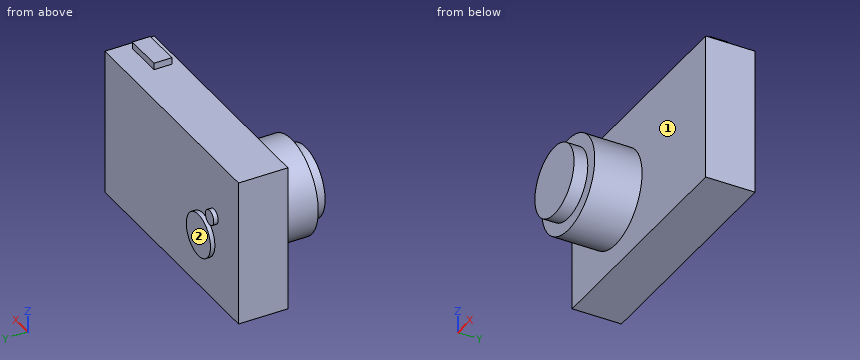
```python
from build123d import *

# Parameters (mm, degrees)
F0_W      = 180.9290349483
F0_H      = 111.6445362568
F1_DEPTH  = 25.4
F2_R      = 35.8615179987
F3_DEPTH  = 35.814
F4_R      = 26.5022456756
F5_DEPTH  = 10.414
F6_W      = 29.163653031
F6_H      = 13.6000299826
F7_DEPTH  = 5.08
F8_DEPTH  = 11.938
F10_R     = 16.3527851641
F10_R_2   = 5.6386158943
F11_DEPTH = 3.302


with BuildPart() as f1:
    # F0 (on Front) → F1 (new body)
    with BuildSketch(Plane.XZ):
        with Locations((-25.5821794271, -14.9854421616)):
            Rectangle(F0_W, F0_H)
    extrude(amount=F1_DEPTH)

    # F2 (on face) → F3 (join)
    with BuildSketch(Plane.XZ.offset(25.4)):
        with Locations((-57.2519302368, -18.0181078613)):
            Circle(F2_R)
    extrude(amount=F3_DEPTH)

    # F4 (on face) → F5 (join)
    with BuildSketch(Plane.XZ.offset(61.214)):
        with Locations((-57.2519302368, -18.0181078613)):
            Circle(F4_R)
    extrude(amount=F5_DEPTH)

    # F6 (on face) → F7 (join)
    with BuildSketch(Plane.XY.offset(40.8368259668)):
        with Locations((44.361977838, -12.2991851531)):
            Rectangle(F6_W, F6_H)
    extrude(amount=F7_DEPTH)

    # F8 (add): a face of the model
    f8_faces = [f1.faces().sort_by_distance(p)[0] for p in [
        (-25.5821794271, 0, -14.9854421616),
    ]]
    extrude(f8_faces, amount=F8_DEPTH)

    # F10 (on face) → F11 (join)
    with BuildSketch(Plane(origin=(0, 11.938, 0), x_dir=(-1, 0, 0), z_dir=(0, 1, 0))):
        with Locations((67.5977021456, -27.2572916001)):
            Circle(F10_R)
        with Locations((82.7291309834, -4.6637952328)):
            Circle(F10_R_2)
    extrude(amount=F11_DEPTH)


solid = f1.part
```
Source: CAD feature listing. Evaluate the final solid. Frame: model axes, mm. Face numbers are marked on the shaded views. A direction names the side the tool comes from. Give positions to 0.01 mm unless a question says otherwise; leave off trailing zeros. Loops run counter-clockwise (first coordinate to the right, second up) from the corner with the lowest first, then second, coordinate; pieces in that order, holes last. Notation, with made-up numbers: (54, 1) -> (103, 1) arc R22 ccw to (103, 35) -> close; hole circle Ø4 at (-6.5, -24.75). An arc over 180 degrees is marked (long way). Use a Markdown table: item, result. Add a question column.
(1) Access query for the marked faces 1 and 2. Directions: +Z, -Z, +X, -X, +Y, -Y. A direction counts if a zero-diameter tool reaches every point of the face in a straight line with its end or side. Return the directions, or none.
(2) Section query C-C (z = 32.5). Output: boundary loops of the cut face in (x, y).
(3) Section query A-A (x = 45). Output: boundary loops of the cut face in (y, z), then the cut area to 3 significant figures.
(4) First-contact query: pin 1 Ø2 at (x, z) = (-81.5, -2.5) entering from -Y; pin 2 Ø18.5 at (x, y) = (9, -2.5) entering from +Z; pin 3 Ø1.5 at (y, z) = (-12.5, 42.5) entering from +X. Flat tips, straight axial feed; report the tip coordinate or a pass-through.
(5) Section query B-B (y = -12). Output: boundary loops of the cut face in (x, z).
(6) Section query D-D (x = -36). Output: boundary loops of the cut face in (y, z).
(7) Ray query, line 1 (Y direction, x = -100.5, z = -29); line 2 (Z direction, x = -95, y = 5); line 3 (Y direction, x = -67.5, z = -4). Return the intervals inside material, ascending.
Checked values:
| question | item | result |
|---|---|---|
| 1 | face 1 | -Y |
| 1 | face 2 | +Z, -Z, +X, -X, +Y |
| 2 | outline | (-116.05, -25.4) -> (64.88, -25.4) -> (64.88, 11.94) -> (-116.05, 11.94) -> close |
| 3 | outline | (-25.4, -70.81) -> (11.94, -70.81) -> (11.94, 40.84) -> (-5.5, 40.84) -> (-5.5, 45.92) -> (-19.1, 45.92) -> (-19.1, 40.84) -> (-25.4, 40.84) -> close |
| 3 | area | 4,240 mm^2 |
| 4 | pin 1 | y = -61.21 |
| 4 | pin 2 | z = 40.84 |
| 4 | pin 3 | x = 58.94 |
| 5 | outline | (-116.05, -70.81) -> (64.88, -70.81) -> (64.88, 40.84) -> (58.94, 40.84) -> (58.94, 45.92) -> (29.78, 45.92) -> (29.78, 40.84) -> (-116.05, 40.84) -> close |
| 6 | outline | (-71.63, -33.85) -> (-61.21, -33.85) -> (-61.21, -46.9) -> (-25.4, -46.9) -> (-25.4, -70.81) -> (11.94, -70.81) -> (11.94, 40.84) -> (-25.4, 40.84) -> (-25.4, 10.87) -> (-61.21, 10.87) -> (-61.21, -2.18) -> (-71.63, -2.18) -> close |
| 7 | line 1 | -25.4 to 11.94 |
| 7 | line 2 | -70.81 to 40.84 |
| 7 | line 3 | -71.63 to 11.94 |
